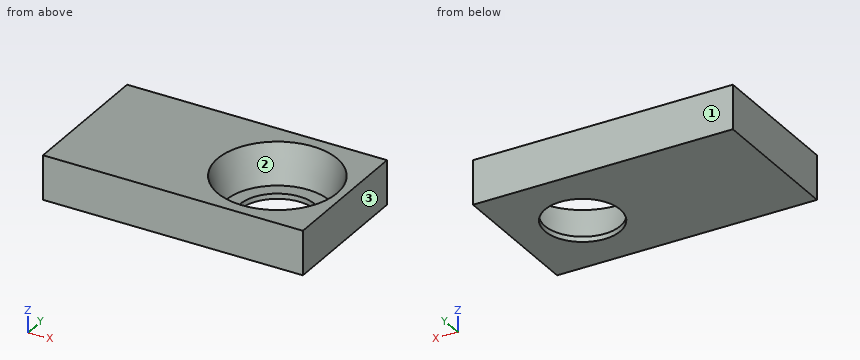
from build123d import *

# Parameters (mm, degrees)
F0_W     = 100
F0_H     = 55
F1_DEPTH = 17
F3_R     = 23
F2_R     = 19.5
F5_R     = 14.5
F5_R_2   = 20.5
F6_DEPTH = 2


with BuildPart() as f1:
    # F0 (on Top) → F1 (new body)
    with BuildSketch(Plane.XY):
        Rectangle(F0_W, F0_H)
    extrude(amount=F1_DEPTH)

    # F3 (on face) → F4 section 0
    with BuildSketch(Plane.XY.offset(17)):
        with Locations((24, 0)):
            Circle(F3_R)
    # F2 (on face) → F4 section 1
    with BuildSketch(Plane(origin=(0, 0, 0), x_dir=(1, 0, 0), z_dir=(0, 0, -1))):
        with Locations((24, 0)):
            Circle(F2_R)
    loft(mode=Mode.SUBTRACT)

    # F5 (on face) → F6 (join)
    with BuildSketch(Plane(origin=(0, 0, 0), x_dir=(1, 0, 0), z_dir=(0, 0, -1))):
        with Locations((24, 0)):
            Circle(F5_R)
        with Locations((24, 0)):
            Circle(F5_R_2)
        with Locations((24, 0)):
            Circle(F5_R, mode=Mode.SUBTRACT)
    extrude(amount=-F6_DEPTH)


solid = f1.part
Here's how the part is built. I have some questions about the finished solid (model axes, mm). Face numbers are marked on the shaded views. Coordinates: 2 decimals unless noted, no trailing zeros. Loops run counter-clockwise (first coordinate to the right, second up) from the corner with the lowest first, then second, coordinate; pieces in that order, holes last.
1. I need wall thicknesses on L1, parallel to Y at x = 24, z = 0.65; L2, parallel to X at y = 0, z = 1; L3, parallel to Y at x = 37.5, z = 14.75. Which ranges of each line are inside material? Lowest first, please.
2. Imagine slicing it at C-C, the plane z = 6. Please give me the cut outline in (x, y).
3. For P1, Ø12, axis at x = 29.5, y = 8, coming from the +Z side, with a flat end and sliding along its axis, tell me the tip position at first contact or that it passes through.
4. Imagine slicing it at A-A, the plane x = 24. Please give me the cut outline in (y, z).
5. Imagine slicing it at B-B, the plane z = 12.75. Please give me the cut outline in (x, y) (3 decimals).
6. If we mould it in two halves opening along Y, with no side actions, what happens to the marked faces 1, 2 and 3? For each: pulls with the +Y half, pulls with the -Y half, needs draft (parallel to the pull), parting line crosses it, or undercut.
Taken from the geometry:
1. L1: y = -27.5 to -14.5, 14.5 to 27.5
1. L2: x = -50 to 9.5, 38.5 to 50
1. L3: y = -27.5 to -18.05, 18.05 to 27.5
2. outline: (-50, -27.5) - (50, -27.5) - (50, 27.5) - (-50, 27.5) - close; hole circle Ø41.47 at (24, 0)
3. P1: stops at z = 2
4. outline: (-27.5, 0) - (-14.5, 0) - (-14.5, 2) - (-19.91, 2) - (-23, 17) - (-27.5, 17) - close; (14.5, 0) - (27.5, 0) - (27.5, 17) - (23, 17) - (19.91, 2) - (14.5, 2) - close
5. outline: (-50, -27.5) - (50, -27.5) - (50, 27.5) - (-50, 27.5) - close; hole circle Ø44.25 at (24, 0)
6. face 1: pulls with the +Y half
6. face 2: undercut
6. face 3: needs draft
